Build history of the part. All positions in model axes, mm. Face numbers are marked on the shaded views. A direction names the side the tool comes from. Round coordinates to 2 decimals unless told otherwise and drop trailing zeros. Order: outer loops, then holes, each group sorted by start corner. A loop starts at its lowest first (then second) coordinate and runs counter-clockwise, first axis right, second up. Notation, with made-up numbers: (67, 68.5) -> (101, 68.5) arc R17 cw to (101, 91.5) -> close; hole circle Ø10 at (46.25, -19). An arc over 180 degrees is marked (long way). Use a Markdown table: item, result. Add a question column.
Item 1: Pin check, flat tips, straight feed: pin 1 (5 mm diameter, centred on x = 9.5, y = 12, fed in from +Z) (3 decimals); pin 2 (2 mm diameter, centred on x = 31, z = 2.5, fed in from +Y); pin 3 (4.5 mm diameter, centred on y = 1, z = 4.5, fed in from +X); pin 4 (2.5 mm diameter, centred on x = 3.91, y = 3.98, fed in from -Z). Stop position of each tip, or through.
Item 2: Slice it at C-C, the plane y = 8.75. State how many separate pieces and enclosed holes the cut face has, plus the area to 3 significant figures.
Item 3: 3-axis set-ups, long thin cutter, end or side, ignore diameter. For the marked faces 3, 4 and 5: which of +Z, -Z, +X, -X, +Y, -Y reach the whole face in a straight line?
Item 4: Slice it at B-B, the plane z = 5.25. Give the cut face in (x, y).
Item 5: Two-plate mould, pull along X, no slides. Class the marked faces 1 and 2: released by +X, released by -X, zero draft, split by the parting line, or undercut.
Item 6: Probe L1, parallel to Y at x = 3.5, z = 3.5; L2, parallel to Z at x = 20.5, y = 0.5; L3, parallel to X at y = 6, z = 2. List the from-to ranges inside material, lowest first.
Item 7: Slice it at A-A, the plane y = 1.5. Give the cut face in (x, z).
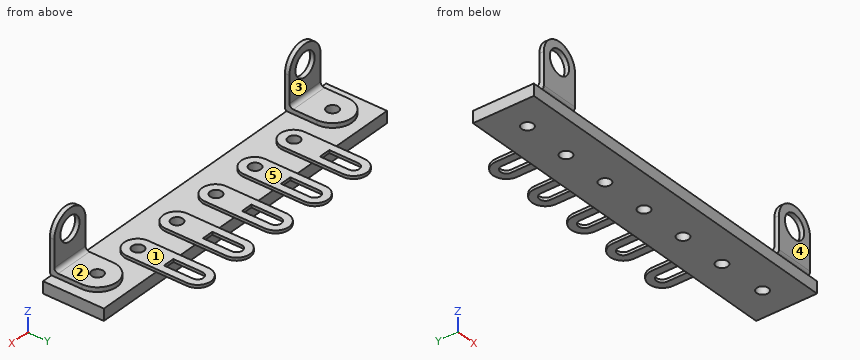
from build123d import *

# Parameters (mm, degrees)
SKETCH1_W           = 46.101
SKETCH1_H           = 7.9502
BASE_EXTRUDE_DEPTH  = 1.524
BOSS_EXTRUDE1_DEPTH = 0.5842
SKETCH3_R           = 1.5621
BOSS_EXTRUDE2_DEPTH = 0.5842
FILLET1_R           = 0.508
SKETCH4_R           = 0.762
CUT_EXTRUDE1_DEPTH  = 48.234733554
MIRROR1_START       = -1
MIRROR1_OUTLINE_R   = 0.762
MIRROR1_DEPTH       = 2.524
MIRROR1_START_2     = 1.524
MIRROR1_2_OUTLINE_R = 0.762
MIRROR1_2_DEPTH     = 0.5842
MIRROR1_START_3     = 1.9304
MIRROR1_3_OUTLINE_W = 5.08
MIRROR1_3_OUTLINE_H = 0.5842
MIRROR1_3_DEPTH     = 2.6034999
MIRROR1_START_4     = 39.6494
MIRROR1_4_DEPTH     = 5.08
MIRROR1_START_5     = -0.2032
MIRROR1_5_OUTLINE_R = 1.5621
MIRROR1_5_DEPTH     = 0.5842
BOSS_EXTRUDE3_DEPTH = 0.381
SKETCH6_R           = 0.762
CUT_EXTRUDE2_DEPTH  = 2.54
LPATTERN1_COUNT     = 5
LPATTERN1_PITCH     = 6.35


with BuildPart() as part:
    # Sketch1 → Base-Extrude (new body)
    with BuildSketch(Plane.XY):
        with Locations((23.0505, 3.9751)):
            Rectangle(SKETCH1_W, SKETCH1_H)
    extrude(amount=BASE_EXTRUDE_DEPTH)

    # Sketch2 → Boss-Extrude1 (add)
    with BuildSketch(Plane.XY.offset(1.524)):
        with BuildLine():
            Line((6.4516, 3.9751), (6.4516, -0.2032))
            Line((6.4516, -0.2032), (1.3716, -0.2032))
            Line((1.3716, -0.2032), (1.3716, 3.9751))
            ThreePointArc((1.3716, 3.9751), (3.9116, 6.5151), (6.4516, 3.9751))
        make_face()
    extrude(amount=BOSS_EXTRUDE1_DEPTH)

    # Sketch3 → Boss-Extrude2 (add)
    with BuildSketch(Plane(origin=(0, -0.2032, 0), x_dir=(-1, 0, 0), z_dir=(0, 1, 0))):
        with BuildLine():
            Line((-1.3716, 6.096), (-1.3716, 1.524))
            Line((-1.3716, 1.524), (-6.4516, 1.524))
            Line((-6.4516, 1.524), (-6.4516, 6.096))
            ThreePointArc((-6.4516, 6.096), (-3.9116, 8.636), (-1.3716, 6.096))
        make_face()
        with Locations(Location((-3.9116, 6.096, 0), (0, 0, 90))):
            Circle(SKETCH3_R, mode=Mode.SUBTRACT)
    extrude(amount=BOSS_EXTRUDE2_DEPTH)

    # Fillet1
    # the kernel refuses this fillet: 0.508 mm, written as the material it adds along each edge
    with BuildSketch(Plane(origin=(6.4516, 0.381, 2.1082), x_dir=(0, 1, 0), z_dir=(-1, 0, 0))) as fillet1_piece_1:
        with BuildLine():
            CenterArc((FILLET1_R, -FILLET1_R), FILLET1_R, 90, 90)
            Line((0, -FILLET1_R), (0, 0))
            Line((0, 0), (FILLET1_R, 0))
        make_face()
    extrude(amount=5.08)
    # the kernel refuses this fillet: 0.508 mm, written as the material it takes off along each edge
    with BuildSketch(Plane(origin=(7.4676, -0.2032, 1.524), x_dir=(0, 1.0, 2.6098982991759982e-11), z_dir=(-1, 0, 0))) as fillet1_2_piece_1:
        with BuildLine():
            CenterArc((0.508, -0.4064), FILLET1_R, 126.869897647, 53.130102355)
            Line((0, -0.4064), (0, 0))
            Line((0, 0), (0.2032, 0))
        make_face()
    extrude(amount=7.112, mode=Mode.SUBTRACT)

    # Sketch4 → Cut-Extrude1 (cut, through all)
    with BuildSketch(Plane.XY.offset(2.1082)):
        with Locations((3.9116, 3.9751)):
            Circle(SKETCH4_R)
    extrude(amount=-CUT_EXTRUDE1_DEPTH, mode=Mode.SUBTRACT)

    # Mirror1: read off the stored shape, not the designer's step
    # Mirror1 outline → Mirror1 (cut)
    with BuildSketch(Plane.XY.offset(MIRROR1_START)):
        with Locations((42.1894, 3.9751)):
            Circle(MIRROR1_OUTLINE_R)
    extrude(amount=MIRROR1_DEPTH, mode=Mode.SUBTRACT)

    # Mirror1 2 outline → Mirror1 2 (add)
    with BuildSketch(Plane.XY.offset(MIRROR1_START_2)):
        with BuildLine():
            Line((39.6494, 3.9751), (39.6494, 0.381))
            Line((39.6494, 0.381), (44.7294, 0.381))
            Line((44.7294, 0.381), (44.7294, 3.9751))
            ThreePointArc((44.7294, 3.9751), (42.1894, 6.5151), (39.6494, 3.9751))
        make_face()
        with Locations((42.1894, 3.9751)):
            Circle(MIRROR1_2_OUTLINE_R, mode=Mode.SUBTRACT)
    extrude(amount=MIRROR1_2_DEPTH)

    # Mirror1 3 outline → Mirror1 3 (add)
    with BuildSketch(Plane.XY.offset(MIRROR1_START_3)):
        with Locations((42.1894, 0.0889)):
            Rectangle(MIRROR1_3_OUTLINE_W, MIRROR1_3_OUTLINE_H)
    extrude(amount=MIRROR1_3_DEPTH)

    # Mirror1 4 outline → Mirror1 4 (add)
    with BuildSketch(Plane.YZ.offset(MIRROR1_START_4)):
        with BuildLine():
            Line((0.381, 1.9304), (-0.2032, 1.9304))
            ThreePointArc((-0.2032, 1.9304), (-0.149569013, 1.703215493), (0, 1.524))
            Line((0, 1.524), (0.381, 1.524))
            Line((0.381, 1.524), (0.381, 1.9304))
        make_face()
        with BuildLine():
            ThreePointArc((0.889, 2.1082), (0.529789755, 2.256989755), (0.381, 2.6162))
            Line((0.381, 2.6162), (0.381, 2.1082))
            Line((0.381, 2.1082), (0.889, 2.1082))
        make_face()
    extrude(amount=MIRROR1_4_DEPTH)

    # Mirror1 5 outline → Mirror1 5 (add)
    with BuildSketch(Plane(origin=(0, 0, 0), x_dir=(1, 0, 0), z_dir=(0, 1, 0)).offset(MIRROR1_START_5)):
        with BuildLine():
            Line((39.6494, -2.6162), (39.6494, -6.096))
            ThreePointArc((39.6494, -6.096), (42.1894, -8.636), (44.7294, -6.096))
            Line((44.7294, -6.096), (44.7294, -2.6162))
            Line((44.7294, -2.6162), (39.6494, -2.6162))
        make_face()
        with Locations((42.1894, -6.096)):
            Circle(MIRROR1_5_OUTLINE_R, mode=Mode.SUBTRACT)
    extrude(amount=MIRROR1_5_DEPTH)

    # Sketch5 → Boss-Extrude3 (add)
    with BuildSketch(Plane.XY.offset(1.524)):
        with BuildLine():
            Line((37.592, 11.9634508), (37.592, 4.128262))
            ThreePointArc((37.592, 4.128262), (35.8394, 2.375662), (34.0868, 4.128262))
            Line((34.0868, 4.128262), (34.0868, 11.9634508))
            ThreePointArc((34.0868, 11.9634508), (35.8394, 13.7160508), (37.592, 11.9634508))
        make_face()
        with BuildLine():
            Line((35.0774, 8.177194519), (36.6014, 8.177194519))
            Line((36.6014, 8.177194519), (36.6014, 11.9634508))
            ThreePointArc((36.6014, 11.9634508), (35.8394, 12.7254508), (35.0774, 11.9634508))
            Line((35.0774, 11.9634508), (35.0774, 8.177194519))
        make_face(mode=Mode.SUBTRACT)
    boss_extrude3 = extrude(amount=BOSS_EXTRUDE3_DEPTH)

    # Sketch6 → Cut-Extrude2 (cut)
    with BuildSketch(Plane.XY.offset(1.905)):
        with Locations((35.8394, 4.1783)):
            Circle(SKETCH6_R)
    cut_extrude2 = extrude(amount=-CUT_EXTRUDE2_DEPTH, mode=Mode.SUBTRACT)

    # LPattern1: Boss-Extrude3, Cut-Extrude2 ×5
    with Locations(*[(-i * LPATTERN1_PITCH, 0, 0) for i in range(1, LPATTERN1_COUNT)]):
        add(boss_extrude3)
        add(cut_extrude2, mode=Mode.SUBTRACT)


solid = part.part
Check sheet entries:
| question | item | result |
|---|---|---|
| 1 | pin 1 | z = 1.905 |
| 1 | pin 2 | y = 13.57 |
| 1 | pin 3 | x = 44.73 |
| 1 | pin 4 | z = 0 |
| 2 | separate pieces | 10 |
| 2 | enclosed holes | 0 |
| 2 | area | 3.77 mm2 |
| 3 | face 3 | +Z, +X, -X, +Y |
| 3 | face 4 | +Z, -Z, +X, -X, -Y |
| 3 | face 5 | +Z, +Y, -Y |
| 4 | outline | (1.37, -0.2) -> (2.6, -0.2) -> (2.6, 0.38) -> (1.37, 0.38) -> close; (5.22, -0.2) -> (6.45, -0.2) -> (6.45, 0.38) -> (5.22, 0.38) -> close; (39.65, -0.2) -> (40.88, -0.2) -> (40.88, 0.38) -> (39.65, 0.38) -> close; (43.5, -0.2) -> (44.73, -0.2) -> (44.73, 0.38) -> (43.5, 0.38) -> close |
| 5 | face 1 | undercut |
| 5 | face 2 | zero draft |
| 6 | L1 | -0.2 to 0.38 |
| 6 | L2 | 0 to 1.52 |
| 6 | L3 | 2.38 to 5.45, 40.66 to 43.72 |
| 7 | outline | (0, 0) -> (46.1, 0) -> (46.1, 1.52) -> (44.73, 1.52) -> (44.73, 2.11) -> (39.65, 2.11) -> (39.65, 1.52) -> (6.45, 1.52) -> (6.45, 2.11) -> (1.37, 2.11) -> (1.37, 1.52) -> (0, 1.52) -> close |
